Autodesk Inventor part; units mm, degrees
ref_plane "Work Plane1" through (0, 0, -40) normal (0, 0, -1) x (1, 0, 0)
ref_plane "YZ Plane" through (0, 0, 0) normal (1, 0, 0) x (0, 1, 0)
ref_plane "XZ Plane" through (0, 0, 0) normal (0, 1, 0) x (-1, 0, 0)
sketch "Sketch1" plane through (0, 0, 0) normal (0, 0, 1) x (1, 0, 0)
  arc A0 (-87.5, 0) -> (87.5, 0) centre (0, 0) ccw
  line L0 (-87.5, 0) -> (87.5, 0) construction
  line L1 (-87.5, -200) -> (87.5, -200)
  line L2 (-87.5, -220) -> (87.5, -220)
  line L3 (-87.5, 0) -> (-107.5, 0)
  line L4 (0, 0) -> (-107, 0)
  line L5 (-107, 0) -> (-107, -200)
  line L6 (-107, -200) -> (-87.5, -200)
  line L7 (-107, -200) -> (-107, -220)
  line L8 (-107, -220) -> (-87.5, -220)
  line L9 (0, 0) -> (107, 0)
  line L10 (107, 0) -> (107, -220)
  line L11 (107, -220) -> (87.5, -220)
  line L12 (87.5, -200) -> (107, -200)
  point P0 (87.5, 0)
  dimension "d0" = 175
  dimension "d1" = 200
  dimension "d9" = 107
  dimension "d10" = 107
  dimension "d13" = 90
  dimension "d15" = 200
  dimension "d17" = 200
  dimension "d18" = 214.5
  dimension "d21" = 20
extrude "Extrusion1" add sketch "Sketch1" along normal blind 20 contours A0 L9 L10 L12 L1 L6 L5 L3
extrude "Extrusion2" add sketch "Sketch1" along normal blind 20 and the other way blind 100 contours L6 L1 L12 L10 L11 L2 L8 L7
ref_plane "Work Plane1" through (0, 0, -40) normal (0, 0, -1) x (1, 0, 0)
mirror "Mirror1" about plane through (0, 0, -40) normal (0, 0, -1) of "Extrusion1"
sketch "Sketch2" plane through (107, 0, 20) normal (1, 0, 0) x (0, 0, -1)
  line L0 (120, -220) -> (0, -220)
  line L1 (0, -220) -> (0, 0)
  line L2 (0, 0) -> (20, 0)
  line L3 (20, -200) -> (20, 0)
  line L4 (20, 0) -> (20, -200)
  line L5 (100, -200) -> (20, -200)
  line L6 (20, -200) -> (100, -200)
  line L7 (100, 0) -> (100, -200)
  line L8 (100, -200) -> (100, 0)
  line L9 (120, -220) -> (120, 0)
  line L10 (100, 0) -> (120, 0)
  line L11 (120, 0) -> (120, -220)
  line L12 (120, -220) -> (0, -220)
extrude "Extrusion3" add sketch "Sketch2" along normal blind 18
properties part number "Support" material "Stainless Steel"
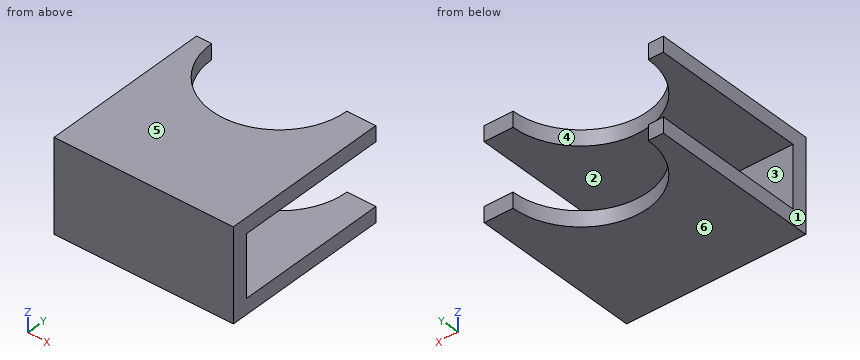
The listing builds one solid part. Answer for the finished solid, in the listing's coordinates (mm). Face numbers are marked on the shaded views. A direction names the side the tool comes from. Give positions to 0.01 mm unless a question says otherwise; leave off trailing zeros. Order: outer loops, then holes, each group sorted by start corner. A loop starts at its lowest first (then second) coordinate and runs counter-clockwise, first axis right, second up.
1) Find section D-D on z = -3.5. Write down the section's boundary in (x, y), then the cut area to 3 significant figures.
Reported:
outline: (-107, -220) - (125, -220) - (125, -200) - (-107, -200) - close
area: 4,640 mm2
2) Consider line 1 along Z through (x, y) = (33, -96); line 2 along Y through (x, z) = (-62.5, -45); line 3 along Y through (x, z) = (17, -87.5). Determine where each line is inside the solid, lowest interval first.
Reported:
line 1: z = -100 to -80, 0 to 20
line 2: y = -220 to -200
line 3: y = -220 to -85.83
3) Find section B-B on x = 109.5. Write down the section's boundary in (y, z), then the cut area to 3 significant figures.
Reported:
outline: (-220, -100) - (0, -100) - (0, -80) - (-200, -80) - (-200, 0) - (0, 0) - (0, 20) - (-220, 20) - close
area: 10,400 mm2
4) Given P1, Ø1.5, axis at x = -28.5, z = -59.5, coming from the +Y side, flat-ended and moving along its own axis, determine where the tip first touches the part or whether it passes through.
Reported:
P1: stops at y = -200
5) Find section C-C on y = -62.5. Write down the section's boundary in (x, z), then the cut area to 3 significant figures.
Reported:
outline: (-107, -100) - (-61.24, -100) - (-61.24, -80) - (-107, -80) - close; (-107, 0) - (-61.24, 0) - (-61.24, 20) - (-107, 20) - close; (61.24, -100) - (125, -100) - (125, -80) - (61.24, -80) - close; (61.24, 0) - (125, 0) - (125, 20) - (61.24, 20) - close
area: 4,380 mm2
6) Determine the mould class of the marked faces 3, 4, 5 and 6 for opening direction Z: pulls with the +Z half, pulls with the -Z half, needs draft (parallel to the pull), parting line crosses it, or undercut.
Reported:
face 3: undercut
face 4: needs draft
face 5: pulls with the +Z half
face 6: pulls with the -Z half
7) Find section A-A on y = -182. Write down the section's boundary in (x, z), then the cut area to 3 significant figures.
Reported:
outline: (-107, -100) - (125, -100) - (125, -80) - (-107, -80) - close; (-107, 0) - (125, 0) - (125, 20) - (-107, 20) - close
area: 9,280 mm2
8) For the marked faces 1 and 2, determine the directions among +Z, -Z, +X, -X, +Y, -Y from which every point of the face is accessible in a straight line to the end or side of a thin tool.
Reported:
face 1: +Z, -Z, -X, +Y, -Y
face 2: +X, -X, +Y
